Part model, mm, in its own coordinate system. A direction names the side the tool comes from. Give positions to 0.01 mm unless a question says otherwise; leave off trailing zeros. Write each loop counter-clockwise with the first axis right and the second up, starting at its lowest first coordinate (ties: lowest second). Pieces come first, ordered by that corner, then holes. Notation, with made-up numbers: M 67.25,18.25 L 72.25,18.25 A11 cw 72.25,31.25 Z; hole C -35.5,74 d10. An arc over 180 degrees is marked long. Use a Markdown table: item, result.
```python
from build123d import *

# Parameters (mm, degrees)
BOSS_EXTRUDE1_DEPTH = 10
CHAMFER1_SIZE       = 5
FILLET1_R           = 5
FILLET2_R           = 7.5
FILLET3_START       = -10
FILLET3_DEPTH       = 20
SKETCH3_R           = 1.625
CUT_EXTRUDE1_DEPTH  = 56.272426005


with BuildPart() as part:
    # Sketch1 → Boss-Extrude1 (new, symmetric)
    with BuildSketch(Plane(origin=(0, 0, 0), x_dir=(0, 0, -1), z_dir=(1, 0, 0))):
        with BuildLine():
            Line((12.319127455, 26), (29.663517642, 26))
            add(Edge.make_bspline(
                [(29.663517642, 26), (29.663517642, 11.740150088), (24.016025287, -2.621570193), (27.532919864, -16.837766109)],
                knots=[0, 0, 0, 0, 1, 1, 1, 1], degree=3))
            Line((27.532919864, -16.837766109), (29.474392891, -16.357471943))
            add(Edge.make_bspline(
                [(31.663517642, 26), (31.663517642, 24.15939465), (31.480704272, 20.46991898), (30.636833768, 13.199740185), (29.144724775, 4.252426008), (28.234715818, -4.480702376), (28.494687407, -11.300478686), (29.06335364, -14.695945165), (29.474392891, -16.357471943)],
                knots=[0, 0, 0, 0, 0.125, 0.25, 0.5, 0.75, 0.875, 1, 1, 1, 1], degree=3))
            Line((31.663517642, 26), (31.663517642, 28))
            Line((31.663517642, 28), (29.663517642, 28))
            Line((29.663517642, 28), (12.319127455, 28))
            Line((12.319127455, 28), (12.319127455, 26))
        make_face()
    extrude(amount=BOSS_EXTRUDE1_DEPTH, both=True)

    # Chamfer1
    chamfer1_edges = [part.edges().sort_by_distance(p)[0] for p in [
        (10, -16.597619026, -28.503656378),
        (-10, -16.597619026, -28.503656378),
        (-10, 27, -12.319127455),
        (10, 27, -12.319127455),
    ]]
    chamfer(chamfer1_edges, length=CHAMFER1_SIZE)

    # Fillet1
    fillet1_edges = [part.edges().sort_by_distance(p)[0] for p in [
        (-5, 26, -29.663517642),
    ]]
    fillet(fillet1_edges, radius=FILLET1_R)

    # Fillet2
    fillet2_edges = [part.edges().sort_by_distance(p)[0] for p in [
        (0, 28, -31.663517642),
    ]]
    fillet(fillet2_edges, radius=FILLET2_R)

    # Fillet3: read off the stored shape, not the designer's step
    # Fillet3 outline → Fillet3 (cut)
    with BuildSketch(Plane.YZ.offset(FILLET3_START)):
        with BuildLine():
            Line((-16.837766109, -27.532919864), (-16.357471943, -29.474392891))
            add(Edge.make_bspline(
                [(-16.357471943, -29.474392891), (-17.106538204, -26.368974262), (-6.635525171, -26.379518895)],
                knots=[0, 0, 0, 1, 1, 1], degree=2, weights=[1, 0.618277336, 1]))
            add(Edge.make_bspline(
                [(-6.635525171, -26.379518895), (-10.042321147, -26.376088146), (-13.444189865, -26.693395004), (-16.837766109, -27.532919864)],
                knots=[0.761288022, 0.761288022, 0.761288022, 0.761288022, 1, 1, 1, 1], degree=3))
        make_face()
    extrude(amount=FILLET3_DEPTH, mode=Mode.SUBTRACT)

    # Sketch3 → Cut-Extrude1 (cut, through all)
    with BuildSketch(Plane(origin=(0, 28, 0), x_dir=(1, 0, 0), z_dir=(0, 1, 0))):
        with Locations(Location((-6.562054303, 18.563874533, 0), (0, 0, 270))):
            Circle(SKETCH3_R)
        with Locations(Location((6.562054303, 18.563874533, 0), (0, 0, 270))):
            Circle(SKETCH3_R)
    extrude(amount=-CUT_EXTRUDE1_DEPTH, mode=Mode.SUBTRACT)


solid = part.part
```
1. Drill centre lines: L1, parallel to Y at x = -4.5, z = -16; L2, parallel to Z at x = 6, y = 23; L3, parallel to Z at x = -0.25, y = -3.5. Where is each one in solid material? Low to high.
Findings below:
| item | result |
|---|---|
| L1 | 26 to 28 |
| L2 | -30.97 to -29.02 |
| L3 | -28.47 to -26.47 |
2. Cut at C-C, the plane z = -14.25. Give the cut face in (x, y).
Findings below:
| item | result |
|---|---|
| outline | M -6.93,26 L 6.93,26 L 6.93,28 L -6.93,28 Z |
3. Tool access for faces 1 (the flat face through (0, 26, -18)), 2 (the flat face through (-10, 11, -29)): list every direction of +Z, -Z, +X, -X, +Y, -Y with a clear straight run to the whole face (end or side of a thin tool).
Findings below:
| item | result |
|---|---|
| face 1 | +Z, +X, -X, -Y |
| face 2 | +Z, -Z, -X, +Y, -Y |
4. Drop flat-ended pins along their axis: P1, Ø2, axis at x = 7, z = -20, coming from the -Y side; P2, Ø12, axis at x = -5, y = 13, coming from the -Z side; P3, Ø1.5, axis at x = 4.5, y = -0.5, coming from the -Z side. Give the stop position or say it passes through.
Findings below:
| item | result |
|---|---|
| P1 | y = 26 |
| P2 | z = -31.29 |
| P3 | z = -28.77 |
5. Cut at B-B, the plane z = -20.75. Give the cut face in (x, y).
Findings below:
| item | result |
|---|---|
| outline | M -10,26 L 10,26 L 10,28 L -10,28 Z |
6. Two-plate mould, pull along X, no slides. Class faces 3 (the flat face through (0, 27, -12.319)), 4 (the cylindrical face through (5.94, 27.014, -17.063)), 5 (the flat face through (7.535, 27.014, -14.854)): released by +X, released by -X, zero draft, split by the parting line, or undercut.
Findings below:
| item | result |
|---|---|
| face 3 | zero draft |
| face 4 | undercut |
| face 5 | released by +X |
7. Cut at A-A, the plane z = -18.25. Give the cut face in (x, y), then the cut area to 3 significant figures.
Findings below:
| item | result |
|---|---|
| outline | M -10,26 L -8.16,26 L -8.16,28 L -10,28 Z; M -4.97,26 L 4.97,26 L 4.97,28 L -4.97,28 Z; M 8.16,26 L 10,26 L 10,28 L 8.16,28 Z |
| area | 27.2 mm2 |
